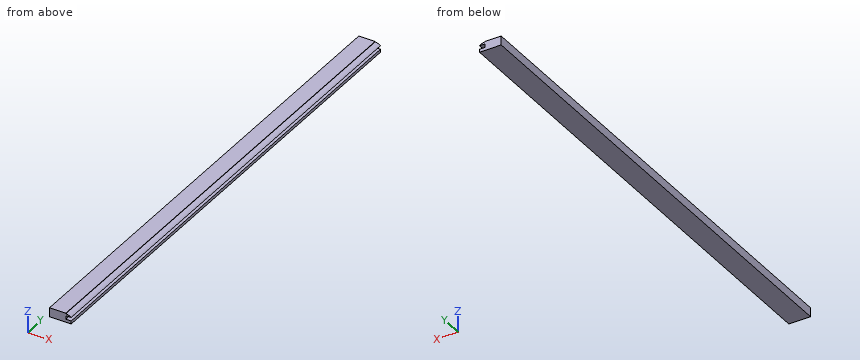
Autodesk Inventor part; units mm, degrees
ref_plane "YZ Plane" through (0, 0, 0) normal (1, 0, 0) x (0, 1, 0)
ref_plane "XZ Plane" through (0, 0, 0) normal (0, 1, 0) x (-1, 0, 0)
ref_plane "XY Plane" through (0, 0, 0) normal (0, 0, 1) x (1, 0, 0)
sketch "Sketch1" plane through (0, 0, 0) normal (0, 1, 0) x (-1, 0, 0)
  line L0 (0, 0) -> (-32.8112, 0)
  line L1 (-38.1, -15.875) -> (0, -15.875)
  line L2 (0, -15.875) -> (0, 0)
  line L3 (0, -15.875) -> (-38.1, -15.875)
  line L4 (-38.1, -15.875) -> (-38.1, -10.5833)
  line L5 (0, -17.5053) -> (0, -15.875)
  line L6 (-28.575, -10.5833) -> (-28.575, -4.2333)
  line L7 (0, -12.2137) -> (0, -17.5053)
  line L8 (-28.575, -4.2333) -> (-38.1, -4.2333)
  line L9 (-38.1, -10.5833) -> (-38.1, -15.875)
  line L10 (-28.575, -10.5833) -> (-38.1, -10.5833)
  line L11 (0, 0) -> (-28.575, 0)
  line L12 (-28.575, 0) -> (-28.575, -0.7937)
  line L13 (-28.575, -0.7937) -> (0, -0.7937)
  line L14 (0, -0.7937) -> (0, 0)
  arc A0 (-28.575, -0.7937) -> (-38.1, -4.2333) centre (-28.575, -15.702) ccw
  dimension "d0" = 38.1
  dimension "d5" = 9.525
  dimension "d6" = 0.7937
  dimension "d10" = 9.525
  dimension "d11" = 28.575
  dimension "d13" = 15.875
  dimension "d14" = 14.9083
  dimension "d15" = 6.35
extrude "Extrusion1" add sketch "Sketch1" along normal blind 876.3
equation "\"d5\" = d10"
properties part number "Cabinet Moulding Long"
The model under review builds one solid part; all positions refer to its coordinate system, in mm. Round coordinates to 2 decimals unless told otherwise and drop trailing zeros. Loops run counter-clockwise (first coordinate to the right, second up) from the corner with the lowest first, then second, coordinate; pieces in that order, holes last. Notation, with made-up numbers: M 29,0 L 81,0 A13 cw 81,11 Z; hole C 76,-8 d3. An arc over 180 degrees is marked long. Write item = value, one per line.
Item 1: Take a section at B-B on z = -6.75. Write out the cut boundary in (x, y) (3 decimals).
Return value:
outline = M 0,0 L 28.575,0 L 28.575,876.3 L 0,876.3 Z
Item 2: For line 1 (X direction, y = 555, z = -10.25) (3 decimals); line 2 (Z direction, x = 29, y = 603) (3 decimals); line 3 (Z direction, x = 36.5, y = 81) (3 decimals), list the stretches that pass through material, from the lowest coordinate up. Write a range as [from, to].
Return value:
line_1 = [0, 28.575]
line_2 = [-15.875, -10.583], [-4.233, -0.8]
line_3 = [-15.875, -10.583], [-4.233, -3.075]
Item 3: Take a section at A-A on y = 139. Write out the cut boundary in (x, z) (3 decimals), then the cut area to 3 significant figures.
Return value:
outline = M 0,-15.875 L 38.1,-15.875 L 38.1,-10.583 L 28.575,-10.583 L 28.575,-4.233 L 38.1,-4.233 A14.908 ccw 28.575,-0.794 L 28.575,0 L 0,0 Z
area = 526 mm2
Item 4: Insertion check: P1, Ø2, axis at x = 31, y = 657.5, coming from the +Z side; P2, Ø3, axis at y = 277, z = -7, coming from the +X side (3 decimals). Each pin has a flat end and moves straight along its axis. Give the tip position at first contact, or say it passes through.
Return value:
P1 = -0.86
P2 = 28.575
